```python
from build123d import *

# Parameters (mm, degrees)
F0_R     = 50
F1_DEPTH = 100
F2_R     = 12.5
F3_DEPTH = 25
F5_D     = 10
F5_DEPTH = 25
F5_TIP   = 3.0043030951
F6_R     = 12.5
F7_DEPTH = 80


with BuildPart() as f1:
    # F0 (on Top) → F1 (new body)
    with BuildSketch(Plane.XY):
        Circle(F0_R)
    extrude(amount=F1_DEPTH)

    # F2 (on face) → F3 (join)
    with BuildSketch(Plane(origin=(0, 0, 0), x_dir=(1, 0, 0), z_dir=(0, 0, -1))):
        Circle(F2_R)
    extrude(amount=F3_DEPTH)

    # F5
    with Locations(Plane(origin=(0, 0, -25), x_dir=(1, 0, 0), z_dir=(0, 0, -1))):
        with Locations((0, 0)):
            Hole(F5_D / 2, depth=F5_DEPTH)
            with Locations((0, 0, -(F5_DEPTH + F5_TIP / 2))):  # 118° drill point
                Cone(0, F5_D / 2, F5_TIP, mode=Mode.SUBTRACT)

    # F6 (on face) → F7 (cut)
    with BuildSketch(Plane.XY.offset(100)):
        with Locations((-30, 0)):
            Circle(F6_R)
        with Locations((0, -30)):
            Circle(F6_R)
        with Locations((30, 0)):
            Circle(F6_R)
        with Locations((0, 30)):
            Circle(F6_R)
    extrude(amount=-F7_DEPTH, mode=Mode.SUBTRACT)


solid = f1.part
```
Verification items for the finished model (mm, model axes). A direction names the side the tool comes from. Give positions to 0.01 mm unless a question says otherwise; leave off trailing zeros. Order: outer loops, then holes, each group sorted by start corner. A loop starts at its lowest first (then second) coordinate and runs counter-clockwise, first axis right, second up. Notation, with made-up numbers: (-2.75, 87.25) -> (51.25, 87.25) arc R7 ccw to (51.25, 94.25) -> close; hole circle Ø2 at (57, -13.5). An arc over 180 degrees is marked (long way). One line per item, written item: value.
(1) Scan lines: line 1 along Y through (x, z) = (0, 74); line 2 along Y through (x, z) = (-7, 90); line 3 along Y through (x, z) = (0, -14). Record each from-to range of solid material in increasing order. Write a range as [from, to].
Final values:
line 1: [-50, -42.5], [-17.5, 17.5], [42.5, 50]
line 2: [-49.51, -40.36], [-19.64, 19.64], [40.36, 49.51]
line 3: [-12.5, -5], [5, 12.5]
(2) Tool access check on faces 5 (the face through (20.08, -7.606, 60.56)), 6 (the face through (-0.2, 5.4, -25)), 7 (the face through (1.08, 4.88, -12.33)). Record the directions out of +Z, -Z, +X, -X, +Y, -Y that give a thin tool (end or side, any length) a straight path to the whole face; none if there is none.
Final values:
face 5: +Z
face 6: -Z, +X, -X, +Y, -Y
face 7: -Z
(3) Gauge pin test, flat ends, axial feed: pin 1 (1.5 mm diameter, centred on y = -26, z = 32, fed in from +X); pin 2 (4 mm diameter, centred on x = 33.5, y = -5.5, fed in from +Z); pin 3 (1.5 mm diameter, centred on x = 38, z = 8, fed in from +Y); pin 4 (10 mm diameter, centred on x = -22.5, y = -4.5, fed in from +Z). Record the tip position at first contact, or that the pin passes through.
Final values:
pin 1: x = 43.16
pin 2: z = 20
pin 3: y = 33.35
pin 4: z = 100
(4) Sectioned sample at A-A on x = 30. Record the cut outline in (y, z), then the cut area to 3 significant figures.
Final values:
outline: (-40, 0) -> (40, 0) -> (40, 100) -> (12.5, 100) -> (12.5, 20) -> (-12.5, 20) -> (-12.5, 100) -> (-40, 100) -> close
area: 6,000 mm^2
(5) Draft check along X on faces 1 (the face through (-0.19, 0.85, 2.48)), 2 (the face through (-1, 1, 100)), 3 (the face through (-2.71, -42.203, 60.56)), 4 (the face through (47.69, 15.02, 49.3)). Enter one of: pulls with the +X half, pulls with the -X half, needs draft (parallel to the pull), parting line crosses it, or undercut.
Final values:
face 1: undercut
face 2: needs draft
face 3: undercut
face 4: parting line crosses it
(6) Sectioned sample at B-B on z = 89.5. Record the cut outline in (x, y), then the cut area to 3 significant figures.
Final values:
outline: circle Ø100 at (0, 0); hole circle Ø25 at (-30, 0); hole circle Ø25 at (0, -30); hole circle Ø25 at (0, 30); hole circle Ø25 at (30, 0)
area: 5,890 mm^2
(7) Sectioned sample at D-D on z = 7. Record the cut outline in (x, y), then the cut area to 3 significant figures.
Final values:
outline: circle Ø100 at (0, 0)
area: 7,850 mm^2
